Source: CAD feature listing. Evaluate the final solid. Frame: model axes, mm. Give positions to 0.01 mm unless a question says otherwise; leave off trailing zeros. Order: outer loops, then holes, each group sorted by start corner. A loop starts at its lowest first (then second) coordinate and runs counter-clockwise, first axis right, second up.
```python
from build123d import *

# Parameters (mm, degrees)
F0_W     = 145
F0_H     = 55
F0_R     = 7.5
F0_R_2   = 1.5
F0_R_3   = 10
F0_R_4   = 4
F1_DEPTH = 3


with BuildPart() as f1:
    # F0 (on Top) → F1 (new body)
    with BuildSketch(Plane.XY):
        with Locations((72.5, -27.5)):
            Rectangle(F0_W, F0_H)
        with Locations((27.5, -42.152297)):
            Circle(F0_R, mode=Mode.SUBTRACT)
        with Locations((57.5, -42.152297)):
            Circle(F0_R, mode=Mode.SUBTRACT)
        with Locations((42, -29.278765)):
            Circle(F0_R_2, mode=Mode.SUBTRACT)
        with Locations((87.5, -42.152297)):
            Circle(F0_R, mode=Mode.SUBTRACT)
        with Locations((117.5, -42.152297)):
            Circle(F0_R, mode=Mode.SUBTRACT)
        with Locations((103, -29.278765)):
            Circle(F0_R_2, mode=Mode.SUBTRACT)
        with Locations((27.5, -17.927479)):
            Circle(F0_R_3, mode=Mode.SUBTRACT)
        with Locations((117.5, -17.927479)):
            Circle(F0_R_3, mode=Mode.SUBTRACT)
        with Locations((72.5, -12.176264)):
            Circle(F0_R_4, mode=Mode.SUBTRACT)
    extrude(amount=F1_DEPTH)


solid = f1.part
```
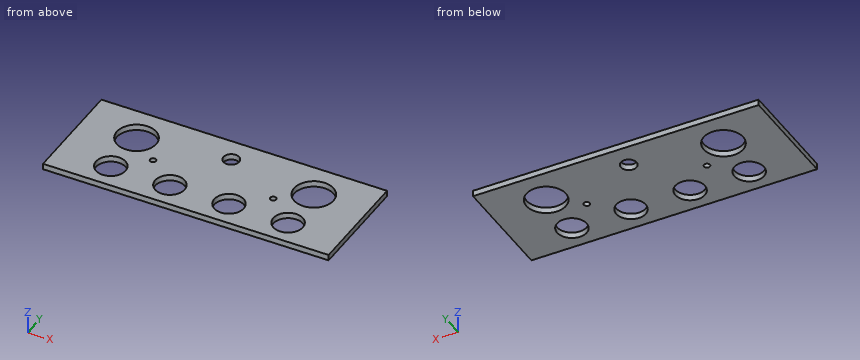
1) Section query C-C, the plane y = -45. Return the cut outline in (x, z).
Report:
outline: (0, 0) - (20.56, 0) - (20.56, 3) - (0, 3) - close; (34.44, 0) - (50.56, 0) - (50.56, 3) - (34.44, 3) - close; (64.44, 0) - (80.56, 0) - (80.56, 3) - (64.44, 3) - close; (94.44, 0) - (110.56, 0) - (110.56, 3) - (94.44, 3) - close; (124.44, 0) - (145, 0) - (145, 3) - (124.44, 3) - close
2) Pin query (flat end, axial travel): pin 1 (12 mm diameter, centred on x = 117.5, y = -17.93, fed in from +Z); pin 2 (13 mm diameter, centred on x = 72.5, y = -12.18, fed in from +Z). Return the tip coordinate at first contact, or that it passes through.
Report:
pin 1: passes through
pin 2: stops at z = 3
3) Section query D-D, the plane z = 1.65. Count the separate pieces of the cut face and the enclosed holes in it, and give its area (3 significant figures).
Report:
separate pieces: 1
enclosed holes: 9
area: 6,580 mm2
4) Material intervals for L1, parallel to Y at x = 27.5, z = 1.3; L2, parallel to Y at x = 103, z = 1.35; L3, parallel to X at y = -37.5, z = 1.95, sorted ascending.
Report:
L1: y = -55 to -49.65, -34.65 to -27.93, -7.93 to 0
L2: y = -55 to -30.78, -27.78 to 0
L3: x = 0 to 21.62, 33.38 to 51.62, 63.38 to 81.62, 93.38 to 111.62, 123.38 to 145
5) Section query B-B, the plane x = 27.5. Return the cut outline in (y, z), and give its area (3 significant figures).
Report:
outline: (-55, 0) - (-49.65, 0) - (-49.65, 3) - (-55, 3) - close; (-34.65, 0) - (-27.93, 0) - (-27.93, 3) - (-34.65, 3) - close; (-7.93, 0) - (0, 0) - (0, 3) - (-7.93, 3) - close
area: 60.0 mm2
6) Section query A-A, the plane x = 57.5. Return the cut outline in (y, z).
Report:
outline: (-55, 0) - (-49.65, 0) - (-49.65, 3) - (-55, 3) - close; (-34.65, 0) - (0, 0) - (0, 3) - (-34.65, 3) - close
